from build123d import *

# Parameters (mm, degrees)
F0_W      = 600
F0_H      = 410
F1_DEPTH  = 5
F3_W      = 5
F3_H      = 410
F4_DEPTH  = 600
F5_W      = 5
F5_H      = 410
F6_DEPTH  = 591
F7_R      = 25
F8_DEPTH  = 25.4
F2_R      = 25
F9_DEPTH  = 25.4
F10_DEPTH = 25.4
F11_DEPTH = 25.4
F2_W      = 5
F2_H      = 410
F12_DEPTH = 21
F13_W     = 5
F13_H     = 410
F14_DEPTH = 495
F15_DEPTH = 76.2
F16_DEPTH = 25.4


with BuildPart() as f1:
    # F0 (on Front) → F1 (new body)
    with BuildSketch(Plane.XZ):
        with Locations((176.868889, 105.440454)):
            Rectangle(F0_W, F0_H)
    extrude(amount=F1_DEPTH)

    # F3 (on face) → F4 (join)
    with BuildSketch(Plane(origin=(0, 0, 0), x_dir=(-1, 0, 0), z_dir=(0, 1, 0))):
        with Locations((-474.368889, 105.440454)):
            Rectangle(F3_W, F3_H)
        with Locations((120.631111, 105.440454)):
            Rectangle(F3_W, F3_H)
    extrude(amount=F4_DEPTH)

    # F5 (on face) → F6 (join)
    with BuildSketch(Plane(origin=(471.868889, 0, 0), x_dir=(0, -1, 0), z_dir=(-1, 0, 0))):
        with Locations((-597.5, 105.440454)):
            Rectangle(F5_W, F5_H)
    extrude(amount=F6_DEPTH)

    # F7 (on face) → F8 (cut)
    with BuildSketch(Plane(origin=(0, 600, 0), x_dir=(-1, 0, 0), z_dir=(0, 1, 0))):
        with Locations((-1.868889, 185.440454)):
            Circle(F7_R)
        with Locations((-243.868889, 185.440454)):
            Circle(F7_R)
    extrude(amount=-F8_DEPTH, mode=Mode.SUBTRACT)

    # F2 (on face) → F9 (cut)
    with BuildSketch(Plane.XZ.offset(5)):
        with Locations((1.868889, 185.440454)):
            Circle(F2_R)
    extrude(amount=-F9_DEPTH, mode=Mode.SUBTRACT)

    # F2 (on face) → F10 (cut)
    with BuildSketch(Plane.XZ.offset(5)):
        with Locations((243.868889, 185.440454)):
            Circle(F2_R)
    extrude(amount=-F10_DEPTH, mode=Mode.SUBTRACT)

    # F2 (on face) → F11 (cut)
    with BuildSketch(Plane.XZ.offset(5)):
        with Locations((1.868889, 5.440454)):
            Circle(F2_R)
    extrude(amount=-F11_DEPTH, mode=Mode.SUBTRACT)

    # F2 (on face) → F12 (join)
    with BuildSketch(Plane.XZ.offset(5)):
        with Locations((-120.631111, 105.440454)):
            Rectangle(F2_W, F2_H)
    extrude(amount=F12_DEPTH)

    # F13 (on face) → F14 (join)
    with BuildSketch(Plane.YZ.offset(-118.131111)):
        with Locations((-23.5, 105.440454)):
            Rectangle(F13_W, F13_H)
    extrude(amount=F14_DEPTH)

    # F2 (on face) → F15 (cut)
    with BuildSketch(Plane.XZ.offset(5)):
        with Locations((1.868889, 5.440454)):
            Circle(F2_R)
    extrude(amount=F15_DEPTH, mode=Mode.SUBTRACT)

    # F2 (on face) → F16 (cut)
    with BuildSketch(Plane.XZ.offset(5)):
        with Locations((159.266515, 43.780868)):
            Circle(F2_R)
    extrude(amount=F16_DEPTH, mode=Mode.SUBTRACT)


solid = f1.part
Geometry: final body of the model. Coordinates: model frame, mm. A direction names the side the tool comes from. Coordinates: 2 decimals unless noted, no trailing zeros. Order: outer loops, then holes, each group sorted by start corner. A loop starts at its lowest first (then second) coordinate and runs counter-clockwise, first axis right, second up.
1) Set-up query: faces 1 (the flat face through (-118.131, -13, 103)), 2 (the cylindrical face through (-17.97, -2.54, -9.77)), 3 (the flat face through (-123.131, 291, 103)), 4 (the flat face through (-118.131, 293, 103)), 5 (the cylindrical face through (268.845, 597.535, 186.54)). Return all of +Z, -Z, +X, -X, +Y, -Y with unobstructed straight access to the full face (end or side cutting, diameter ignored); none if empty.
Result sheet:
face 1: +Z, -Z, +X
face 2: -Y
face 3: +Z, -Z, -X, +Y, -Y
face 4: +Z, -Z
face 5: +Y
2) First-contact query: P1, Ø4, axis at y = -23.5, z = 90.5, coming from the +X side. Flat tip, straight axial feed; report the tip coordinate or a pass-through.
Result sheet:
P1: stops at x = 376.87
3) Section D-D (z = 176). Return loops of the section in (x, y).
Result sheet:
outline: (-123.13, -26) - (376.87, -26) - (376.87, -21) - (-118.13, -21) - (-118.13, -5) - (-21.28, -5) - (-21.28, 0) - (-118.13, 0) - (-118.13, 595) - (-21.28, 595) - (-21.28, 600) - (-123.13, 600) - close; (25.02, -5) - (220.72, -5) - (220.72, 0) - (25.02, 0) - close; (25.02, 595) - (220.72, 595) - (220.72, 600) - (25.02, 600) - close; (267.02, -5) - (476.87, -5) - (476.87, 600) - (267.02, 600) - (267.02, 595) - (471.87, 595) - (471.87, 0) - (267.02, 0) - close
4) Ray query, probe 1 along Y at (x, z) = (182, -72); probe 2 along X at (y, z) = (348.5, 165.5); probe 3 along Y at (x, z) = (143.5, 58). Return the intervals inside material, ascending.
Result sheet:
probe 1: y = -26 to -21, -5 to 0, 595 to 600
probe 2: x = -123.13 to -118.13, 471.87 to 476.87
probe 3: y = -5 to 0, 595 to 600
5) Section A-A (z = -35). Return loops of the section in (x, y).
Result sheet:
outline: (-123.13, -26) - (376.87, -26) - (376.87, -21) - (-118.13, -21) - (-118.13, -5) - (476.87, -5) - (476.87, 600) - (-123.13, 600) - close; hole (-118.13, 0) - (471.87, 0) - (471.87, 595) - (-118.13, 595) - close
6) Section B-B (y = 540). Return loops of the section in (x, z), then the cut area to 3 significant figures.
Result sheet:
outline: (-123.13, -99.56) - (-118.13, -99.56) - (-118.13, 310.44) - (-123.13, 310.44) - close; (471.87, -99.56) - (476.87, -99.56) - (476.87, 310.44) - (471.87, 310.44) - close
area: 4,100 mm2
7) Draft query along X for faces 6 (the flat face through (476.869, 293, 103)), 7 (the flat face through (123, -26, 103)), 8 (the cylindrical face through (240.614, -2.535, 210.228)), 9 (the cylindrical face through (-17.97, -23.46, -9.77)). Return one class per face: released by +X, released by -X, zero draft, split by the parting line, or undercut.
Result sheet:
face 6: released by +X
face 7: zero draft
face 8: undercut
face 9: undercut
8) Section C-C (x = 124.5). Return loops of the section in (y, z).
Result sheet:
outline: (-26, -99.56) - (-21, -99.56) - (-21, 310.44) - (-26, 310.44) - close; (-5, -99.56) - (0, -99.56) - (0, 310.44) - (-5, 310.44) - close; (595, -99.56) - (600, -99.56) - (600, 310.44) - (595, 310.44) - close
